Source: CAD feature listing. Evaluate the final solid. Frame: model axes, mm. A direction names the side the tool comes from. Coordinates: 2 decimals unless noted, no trailing zeros. Write each loop counter-clockwise with the first axis right and the second up, starting at its lowest first coordinate (ties: lowest second). Pieces come first, ordered by that corner, then holes. Notation, with made-up numbers: (-28.5, 18.25) -> (-10.5, 18.25) arc R17 ccw to (-10.5, 32.25) -> close; hole circle Ø5 at (53.5, 30.5). An arc over 180 degrees is marked (long way). Write item = value, one per line.
from build123d import *

# Parameters (mm, degrees)
F0_R     = 22.225
F0_R_2   = 17.4625
F1_DEPTH = 12.7
F4_R     = 21.498416
F4_R_2   = 6.818861
F5_DEPTH = 12.7


with BuildPart() as f1:
    # F0 (on Front) → F1 (new body)
    with BuildSketch(Plane.XZ):
        Circle(F0_R)
        Circle(F0_R_2, mode=Mode.SUBTRACT)
    extrude(amount=F1_DEPTH)

    # F2 (on Right) → F3 (revolve)
    with BuildSketch(Plane.YZ):
        Polygon((-25.4, 7.9375), (-12.7, 16.581038), (-12.7, 21.541582), (-25.4, 21.541582), align=None)
    revolve(axis=Axis((0, -12.7, 0), (0, -1, 0)))

    # F4 (on face) → F5 (join)
    with BuildSketch(Plane.XZ.offset(25.4)):
        Circle(F4_R)
        Circle(F4_R_2, mode=Mode.SUBTRACT)
    extrude(amount=F5_DEPTH)


solid = f1.part
1) Reachability of faces 4 (the flat face through (14.15, -12.7, -8.97)), 5 (the cylindrical face through (-1.478, -31.661, -6.657)), 6 (the cylindrical face through (13.1, -19.1, -17.1)) from +Z, -Z, +X, -X, +Y, -Y: full face, straight path, thin tool, end or side. Return the list, or none.
Answer block:
face_4 = +Y
face_5 = +Y, -Y
face_6 = -Y
2) Material intervals for probe 1 along Z at (x, y) = (0, -7) (1 decimal); probe 2 along Z at (x, y) = (0, -30.25); probe 3 along Y at (x, z) = (-12, 12), sorted ascending. Write a range as [from, to].
Answer block:
probe_1 = [-22.2, -17.5], [17.5, 22.2]
probe_2 = [-21.5, -6.82], [6.82, 21.5]
probe_3 = [-38.1, -12.7]
3) First-contact query: pin 1 Ø12.5 at (x, z) = (-3, 1.5) entering from +Y; pin 2 Ø11 at (x, z) = (0, 0) entering from +Y; pin 3 Ø8 at (x, y) = (13.5, -31) entering from -Z; pin 4 Ø5 at (x, z) = (13, 16.5) entering from +Y. Flat tips, straight axial feed; report the tip coordinate or a pass-through.
Answer block:
pin_1 = -22.95
pin_2 = through
pin_3 = -19.29
pin_4 = 0
4) Pull-direction query (X, two-part tool) for faces 1 (the cylindrical face through (21.199, -6.261, 6.676)), 2 (the flat face through (10, 0, -15)), 3 (the conical face through (8.277, -24.606, -1.838)); classes: +X half, -X half, draft (parallel to the pull), parting line (faces both ways), or undercut.
Answer block:
face_1 = parting line
face_2 = draft
face_3 = undercut
5) Cut plane D-D, the plane x = 19. Output: boundary loops of the cut face in (y, z).
Answer block:
outline = (-38.1, -10.06) -> (-25.4, -10.06) -> (-25.4, -10.15) -> (-12.7, -10.15) -> (-12.7, -11.53) -> (0, -11.53) -> (0, 11.53) -> (-12.7, 11.53) -> (-12.7, 10.15) -> (-25.4, 10.15) -> (-25.4, 10.06) -> (-38.1, 10.06) -> close
